Can you work these out from the model? Positions are in its coordinate system, mm. Face numbers are marked on the shaded views. A direction names the side the tool comes from. Give positions to 0.01 mm unless a question says otherwise; leave off trailing zeros. Loops run counter-clockwise (first coordinate to the right, second up) from the corner with the lowest first, then second, coordinate; pieces in that order, holes last. Notation, with made-up numbers: (3.5, 5.25) - (24.5, 5.25) arc R26 ccw to (24.5, 39.25) - close; hole circle Ø8 at (-31.5, 68.25). An arc over 180 degrees is marked (long way). Answer as a JSON object with one key per item and string values.
```python
from build123d import *

# Parameters (mm, degrees)
CUT_EXTRUDE_1_REACH      = 22.18
CUT_EXTRUDE_1_END_RADIUS = 1.5


with BuildPart() as part:
    # 草图2 → 旋转1 (revolve)
    with BuildSketch(Plane.XY, mode=Mode.PRIVATE) as revolve_1_sk:
        Polygon((1.5, 14), (6.5, 14), (6.5, 13), (4.75, 13), (4.75, 6), (6.5, 6), (6.5, 0), (1.5, 0), align=None)
    revolve(revolve_1_sk.sketch.rotate(Axis((0, 66, 0), (0, -1, 0)), 90), axis=Axis((0, 66, 0), (0, -1, 0)))

    # 切除-拉伸1: up to this cylinder (the profile starts outside it)
    cut_extrude_1_end = Plane(origin=(0, 3, 0), z_dir=(0, 1, 0)) * Cylinder(CUT_EXTRUDE_1_END_RADIUS, 48.36, mode=Mode.PRIVATE)
    # 草图3 → 切除-拉伸1 (cut, up to the surface)
    with BuildSketch(Plane.XY.offset(6.5), mode=Mode.PRIVATE) as cut_extrude_1_sk1:
        with BuildLine():
            ThreePointArc((1.5, 3), (1.060660172, 4.060660172), (0, 4.5))
            Line((0, 4.5), (0, 1.5))
            ThreePointArc((0, 1.5), (1.060660172, 1.939339828), (1.5, 3))
        make_face()
    cut_extrude_1_tool1 = extrude(cut_extrude_1_sk1.sketch, amount=-CUT_EXTRUDE_1_REACH, mode=Mode.PRIVATE) - cut_extrude_1_end
    add(cut_extrude_1_tool1.solids().sort_by_distance((0.63662, 3, 6.5))[0], mode=Mode.SUBTRACT)
    # 草图3 → 切除-拉伸1 (cut, up to the surface)
    with BuildSketch(Plane.XY.offset(6.5), mode=Mode.PRIVATE) as cut_extrude_1_sk2:
        with BuildLine():
            Line((0, 1.5), (0, 4.5))
            ThreePointArc((0, 4.5), (-1.5, 3), (0, 1.5))
        make_face()
    cut_extrude_1_tool2 = extrude(cut_extrude_1_sk2.sketch, amount=-CUT_EXTRUDE_1_REACH, mode=Mode.PRIVATE) - cut_extrude_1_end
    add(cut_extrude_1_tool2.solids().sort_by_distance((-0.63662, 3, 6.5))[0], mode=Mode.SUBTRACT)
    # 草图3 → 切除-拉伸1 (cut, up to the surface)
    with BuildSketch(Plane.XY.offset(6.5), mode=Mode.PRIVATE) as cut_extrude_1_sk3:
        with BuildLine():
            ThreePointArc((1.5, 3), (1.060660172, 4.060660172), (0, 4.5))
            Line((0, 4.5), (0, 1.5))
            ThreePointArc((0, 1.5), (1.060660172, 1.939339828), (1.5, 3))
        make_face()
    cut_extrude_1_tool3 = extrude(cut_extrude_1_sk3.sketch, amount=-CUT_EXTRUDE_1_REACH, mode=Mode.PRIVATE) - cut_extrude_1_end
    add(cut_extrude_1_tool3.solids().sort_by_distance((0.63662, 3, 6.5))[0], mode=Mode.SUBTRACT)
    # 草图3 → 切除-拉伸1 (cut, up to the surface)
    with BuildSketch(Plane.XY.offset(6.5), mode=Mode.PRIVATE) as cut_extrude_1_sk4:
        with BuildLine():
            Line((0, 1.5), (0, 4.5))
            ThreePointArc((0, 4.5), (-1.5, 3), (0, 1.5))
        make_face()
    cut_extrude_1_tool4 = extrude(cut_extrude_1_sk4.sketch, amount=-CUT_EXTRUDE_1_REACH, mode=Mode.PRIVATE) - cut_extrude_1_end
    add(cut_extrude_1_tool4.solids().sort_by_distance((-0.63662, 3, 6.5))[0], mode=Mode.SUBTRACT)


solid = part.part
```
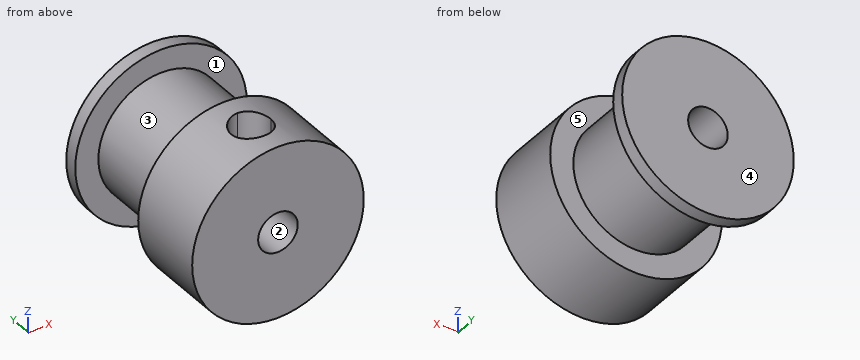
1) I need wall thicknesses on L1, parallel to X at y = 10, z = 0; L2, parallel to Y at x = 6, z = -1.75; L3, parallel to Y at x = -0.25, z = 5.5. Which ranges of each line are inside material? Lowest first, please.
Check sheet entries:
{"L1": "-4.75 to -1.5, 1.5 to 4.75", "L2": "0 to 6, 13 to 14", "L3": "0 to 1.52, 4.48 to 6, 13 to 14"}
2) Imagine slicing it at A-A on x = 5.75. Write out the boundary of the cut face in (y, z), and give its area (3 significant figures).
Check sheet entries:
{"outline": "(0, -3.03) - (6, -3.03) - (6, 3.03) - (0, 3.03) - close; (13, -3.03) - (14, -3.03) - (14, 3.03) - (13, 3.03) - close", "area": "42.4 mm2"}
3) Imagine slicing it at B-B on x = -1. Write out the boundary of the cut face in (y, z).
Check sheet entries:
{"outline": "(0, -6.42) - (6, -6.42) - (6, -4.64) - (13, -4.64) - (13, -6.42) - (14, -6.42) - (14, -1.12) - (0, -1.12) - close; (0, 1.12) - (1.88, 1.12) - (1.88, 6.42) - (0, 6.42) - close; (4.12, 1.12) - (14, 1.12) - (14, 6.42) - (13, 6.42) - (13, 4.64) - (6, 4.64) - (6, 6.42) - (4.12, 6.42) - close"}
4) If we mould it in two halves opening along X, with no side actions, what happens to the marked faces 1, 2 and 3? For each: released by +X, released by -X, zero draft, split by the parting line, or undercut.
Check sheet entries:
{"face 1": "zero draft", "face 2": "undercut", "face 3": "split by the parting line"}
5) Imagine slicing it at D-D on z = -4. Write out the boundary of the cut face in (x, y), and give its area (3 significant figures).
Check sheet entries:
{"outline": "(-5.12, 0) - (5.12, 0) - (5.12, 6) - (2.56, 6) - (2.56, 13) - (5.12, 13) - (5.12, 14) - (-5.12, 14) - (-5.12, 13) - (-2.56, 13) - (-2.56, 6) - (-5.12, 6) - close", "area": "108 mm2"}
6) Which directions (+Z, -Z, +X, -X, +Y, -Y) give clear straight access to the entire face, cutting with the end or side of a thin tool? Please do the marked faces 4 and 5.
Check sheet entries:
{"face 4": "+Z, -Z, +X, -X, +Y", "face 5": "none"}
7) Imagine slicing it at C-C on y = 9.75. Write out the boundary of the cut face in (x, z), and give its area (3 significant figures).
Check sheet entries:
{"outline": "circle Ø9.5 at (0, 0); hole circle Ø3 at (0, 0)", "area": "63.8 mm2"}
8) I'm going to push flat-ended pins straight in: P1, Ø4, axis at x = -2, z = -1, coming from the -Y side; P2, Ø4, axis at x = -1.5, y = 8.5, coming from the -Z side; P3, Ø2, axis at x = 4.5, y = 6, coming from the +Z side; P4, Ø1, axis at x = 4.5, y = 6, coming from the -Z side. Where does each tip first touch, or does it pass through?
Check sheet entries:
{"P1": "y = 0", "P2": "z = -4.75", "P3": "z = 5.48", "P4": "z = -5.12"}
